The drawing under review shows one solid part. Ordinate dimensions are in mm from its lowest x, y, z. A direction names the side the tool comes from. Give positions to 0.01 mm unless a question says otherwise; leave off trailing zeros. Write each loop counter-clockwise with the first axis right and the second up, starting at its lowest first coordinate (ties: lowest second). Pieces come first, ordered by that corner, then holes.
Q1. Insertion check: P1, Ø12, axis at y = 50, z = 2.5, coming from the +X side; P2, Ø4.5, axis at y = 1.5, z = 13, coming from the -X side; P3, Ø3.5, axis at x = 4.5, z = 11.5, coming from the +Y side. Each pin has a flat end and moves straight along its axis. Give the tip position at first contact, or say it passes through.
Q2. We need section D-D (z = 10). Give the number of separate pieces and of enclosed holes in the cut face, then the cut area to 3 significant figures.
Q3. Machinability: for the marked faces 1, 2 and 3, which of the approach directions +Z, -Z, +X, -X, +Y, -Y give a long, thin tool a straight path to every point of the face, cutting with its end or side? Answer none if there is none.
Q4. We need section B-B (y = 58). Write out the cut boundary in (x, z).
Q5. We need section C-C (z = 3.25). Write out the cut boundary in (x, y), then the cut area to 3 significant figures.
Q6. We need section A-A (x = 127.5). Write out the cut boundary in (y, z), then the cut area to 3 significant figures.
Q7. Mouldability with a two-part tool opening along Y and no side actions: class the marked faces 4, 5 and 6 as released by +Y, released by -Y, zero draft, split by the parting line, or undercut.
Q8. For line 1 (Y direction, x = 139, z = 6.25); line 2 (Z direction, x = 154, y = 82); line 3 (Y direction, x = 8.1, z = 10), list the stretches that pass through material, from the lowest coordinate up.
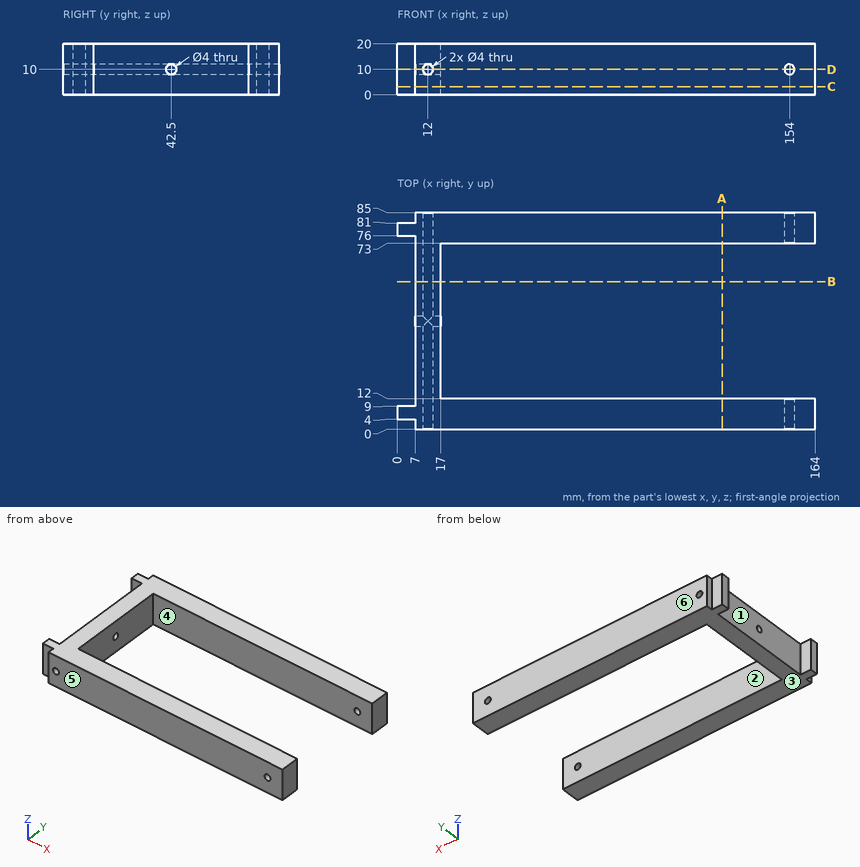
Computed:
1. P1: stops at x = 17
1. P2: stops at x = 7
1. P3: stops at y = 81
2. separate pieces: 6
2. enclosed holes: 0
2. area: 3,990 mm2
3. face 1: +Z, -Z, -X
3. face 2: +Z, -Z, +X
3. face 3: -Z, +X, -X, +Y, -Y
4. outline: (7, 0) - (17, 0) - (17, 20) - (7, 20) - close; hole circle Ø4 at (12, 10)
5. outline: (0, 4) - (7, 4) - (7, 0) - (164, 0) - (164, 12) - (17, 12) - (17, 73) - (164, 73) - (164, 85) - (7, 85) - (7, 81) - (0, 81) - (0, 76) - (7, 76) - (7, 9) - (0, 9) - close
5. area: 4,450 mm2
6. outline: (0, 0) - (12, 0) - (12, 20) - (0, 20) - close; (73, 0) - (85, 0) - (85, 20) - (73, 20) - close
6. area: 480 mm2
7. face 4: undercut
7. face 5: released by -Y
7. face 6: released by +Y
8. line 1: y = 0 to 12, 73 to 85
8. line 2: z = 0 to 8, 12 to 20
8. line 3: y = 0 to 40.5, 44.5 to 85
